```python
from build123d import *

# Parameters (mm, degrees)
SKETCH1_R           = 65
SKETCH1_R_2         = 2.525
SKETCH1_R_3         = 55
BOSS_EXTRUDE1_DEPTH = 65
SKETCH2_R           = 9.525
CUT_EXTRUDE1_DEPTH  = 113.583302492
SKETCH3_W           = 64
SKETCH3_H           = 58.3
CUT_EXTRUDE2_DEPTH  = 113.583302665


with BuildPart() as part:
    # Sketch1 → Boss-Extrude1 (new body)
    with BuildSketch(Plane(origin=(0, 0, 0), x_dir=(1, 0, 0), z_dir=(0, 1, 0))):
        with Locations(Location((0, 0, 0), (0, 0, 270))):
            Circle(SKETCH1_R)
        with Locations(Location((0, 60, 0), (0, 0, 270))):
            Circle(SKETCH1_R_2, mode=Mode.SUBTRACT)
        with Locations(Location((60, 0, 0), (0, 0, 270))):
            Circle(SKETCH1_R_2, mode=Mode.SUBTRACT)
        with Locations(Location((0, -60, 0), (0, 0, 270))):
            Circle(SKETCH1_R_2, mode=Mode.SUBTRACT)
        with Locations(Location((-60, 0, 0), (0, 0, 270))):
            Circle(SKETCH1_R_2, mode=Mode.SUBTRACT)
        with Locations(Location((0, 0, 0), (0, 0, 270))):
            Circle(SKETCH1_R_3, mode=Mode.SUBTRACT)
    extrude(amount=BOSS_EXTRUDE1_DEPTH)

    # Sketch2 → Cut-Extrude1 (cut, through all)
    with BuildSketch(Plane(origin=(0, 0, 0), x_dir=(0, 0, -1), z_dir=(1, 0, 0))):
        with Locations(Location((-24.25, 30, 0), (0, 0, 180))):
            Circle(SKETCH2_R)
    extrude(amount=CUT_EXTRUDE1_DEPTH, mode=Mode.SUBTRACT)

    # Sketch3 → Cut-Extrude2 (cut, through all)
    with BuildSketch(Plane(origin=(0, 0, 0), x_dir=(0, 0, -1), z_dir=(1, 0, 0))):
        with Locations((-23, 30)):
            Rectangle(SKETCH3_W, SKETCH3_H)
        with BuildLine():
            Line((-41.625, 43.85), (-41.625, 53.85))
            ThreePointArc((-41.625, 53.85), (-44.875, 57.1), (-48.125, 53.85))
            Line((-48.125, 53.85), (-48.125, 43.85))
            ThreePointArc((-48.125, 43.85), (-44.875, 40.6), (-41.625, 43.85))
        make_face(mode=Mode.SUBTRACT)
        with BuildLine():
            Line((2.125, 43.85), (2.125, 53.85))
            ThreePointArc((2.125, 53.85), (-1.125, 57.1), (-4.375, 53.85))
            Line((-4.375, 53.85), (-4.375, 43.85))
            ThreePointArc((-4.375, 43.85), (-1.125, 40.6), (2.125, 43.85))
        make_face(mode=Mode.SUBTRACT)
    extrude(amount=CUT_EXTRUDE2_DEPTH, mode=Mode.SUBTRACT)


with BuildPart() as cut_extrude2_kept_piece:
    # of the separate pieces the step leaves, the one the design keeps (cut_extrude2_pieces_kept)
    add(part.part.solids().sort_by_distance((0, 0, 65))[0])


solid = cut_extrude2_kept_piece.part
```
Verification items for the finished model (mm, model axes). A direction names the side the tool comes from. Coordinates: 2 decimals unless noted, no trailing zeros. Order: outer loops, then holes, each group sorted by start corner. A loop starts at its lowest first (then second) coordinate and runs counter-clockwise, first axis right, second up. Notation, with made-up numbers: (72.5, 34) -> (99.5, 34) arc R29 cw to (99.5, 54) -> close; hole circle Ø1 at (15, -32). An arc over 180 degrees is marked (long way). Put each result on its own line as item: value. Start each with the question number.
1) Go/stop test with flat-tipped pins: pin 1 (10 mm diameter, centred on y = 27.5, z = 5, fed in from -X); pin 2 (5 mm diameter, centred on x = 57, y = 41.5, fed in from +Z); pin 3 (6 mm diameter, centred on x = 60, z = 0, fed in from +Y); pin 4 (4.5 mm diameter, centred on x = -60, z = 0, fed in from +Y). Record where each tip stops, or that it passes through.
2) Cross-section at A-A (x = -60). Enter the section's corners in (y, z) (3 decimals).
3) Cross-section at B-B (x = 60). Enter the section's corners in (y, z) (3 decimals).
4) Release check for a two-part mould opening along Z. For faces 1 (the cylindrical face through (-62.24, 32.045, 1.165)), 2 (the cylindrical face through (-63.454, 32.045, -14.091)), 3 (the flat face through (53.3, 65, -14.7)) record: pulls with the +Z half, pulls with the -Z half, needs draft (parallel to the pull), parting line crosses it, or undercut.
5) Cross-section at C-C (z = 60). Enter the section's corners in (x, y) (3 decimals).
6) Tool access check on faces 4 (the cylindrical face through (57.76, 62.034, 1.165)), 5 (the flat face through (59, 30, -9)), 6 (the flat face through (49, 0.85, 28)). Record the directions out of +Z, -Z, +X, -X, +Y, -Y that give a thin tool (end or side, any length) a straight path to the whole face; none if there is none.
7) Cross-section at D-D (y = 50.5). Enter the section's corners in (x, z) (3 decimals), plus the area to 3 significant figures.
8) Material ranges on L1, parallel to X at y = 30.5, z = 0 (3 decimals); L2, parallel to Y at x = 37.5, z = 42; L3, parallel to Z at x = 30.5, y = 16, recorded low to high.
Geometry check:
1. pin 1: stops at x = -65
1. pin 2: stops at z = -9
1. pin 3: stops at y = 65
1. pin 4: passes through
2. outline: (0, -25) -> (65, -25) -> (65, -2.525) -> (0, -2.525) -> close; (0, 2.525) -> (65, 2.525) -> (65, 25) -> (0, 25) -> close
3. outline: (0, -25) -> (65, -25) -> (65, -2.525) -> (59.15, -2.525) -> (59.15, -9) -> (0.85, -9) -> (0.85, -2.525) -> (0, -2.525) -> close; (0, 2.525) -> (0.85, 2.525) -> (0.85, 25) -> (0, 25) -> close; (59.15, 2.525) -> (65, 2.525) -> (65, 25) -> (59.15, 25) -> close
4. face 1: undercut
4. face 2: parting line crosses it
4. face 3: needs draft
5. outline: (-25, 0) -> (-2.525, 0) -> (-2.525, 65) -> (-25, 65) -> close; (2.525, 0) -> (25, 0) -> (25, 65) -> (2.525, 65) -> close
6. face 4: +Y, -Y
6. face 5: +Z, +X
6. face 6: +X
7. outline: (0, 55) -> (34.641, 55) arc R65 ccw (long way) to (64.374, -9) -> (54.259, -9) arc R55 cw (long way) to start; hole circle Ø5.05 at (-60, 0); hole circle Ø5.05 at (0, -60); hole circle Ø5.05 at (0, 60)
7. area: 2,910 mm^2
8. L1: x = -65 to -62.525, -57.475 to -55
8. L2: y = 0 to 0.85, 59.15 to 65
8. L3: z = -57.4 to -45.77, 55 to 57.4
